Check sheet for the drawn part. Datum: minimum x, y, z corner. Units: mm. A direction names the side the tool comes from. Give positions to 0.01 mm unless a question says otherwise; leave off trailing zeros. Loops run counter-clockwise (first coordinate to the right, second up) from the corner with the lowest first, then second, coordinate; pieces in that order, holes last. Notation, with made-up numbers: (-24, 82) - (-8, 82) arc R24 ccw to (-8, 101) - close; hole circle Ø10 at (62.5, 73). An arc over 180 degrees is marked (long way). Answer in a Markdown table with one row per item.
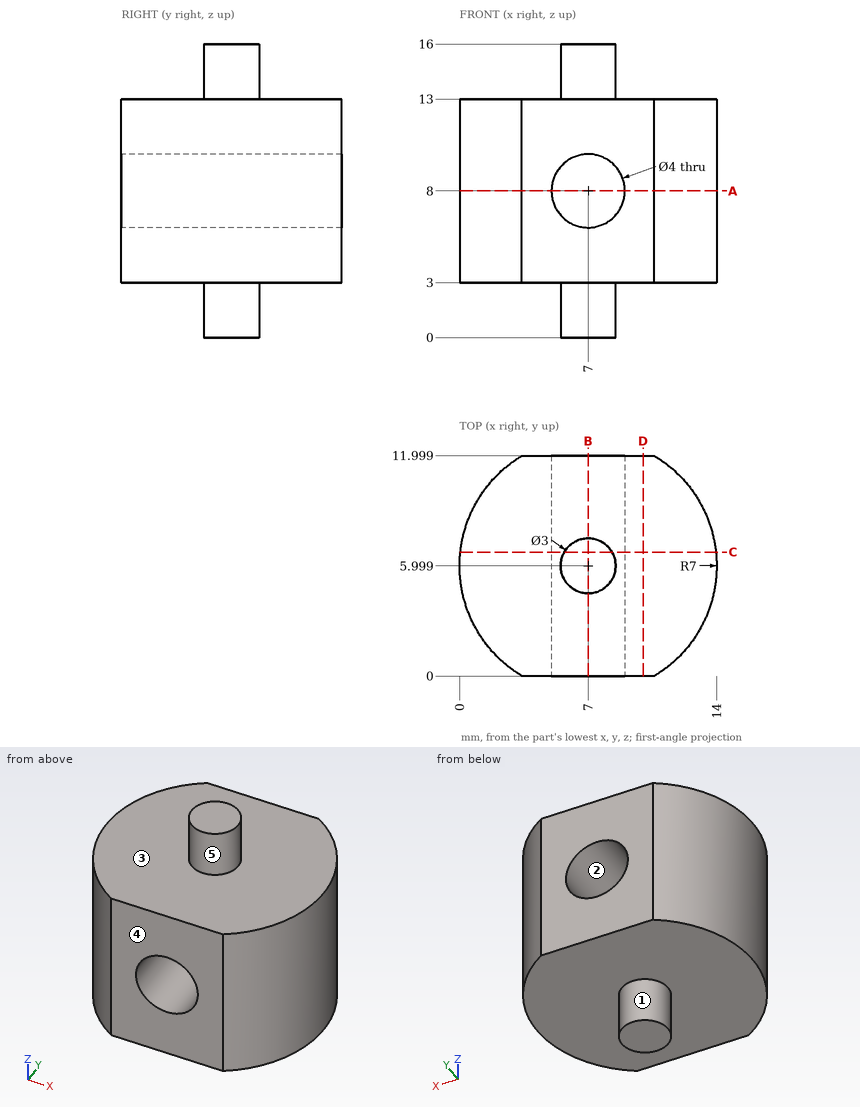
Q1. Draft check along Z on the marked faces 1, 2 and 3. Enter one of: +Z half, -Z half, draft (parallel to the pull), parting line (faces both ways), or undercut.
Completed:
| item | result |
|---|---|
| face 1 | draft |
| face 2 | undercut |
| face 3 | +Z half |
Q2. Sectioned sample at D-D (x = 10). Record the cut outline in (y, z), and give its area (3 significant figures).
Completed:
| item | result |
|---|---|
| outline | (0, 3) - (12, 3) - (12, 13) - (0, 13) - close |
| area | 120 mm^2 |
Q3. Thickness scan on line 1 (Z direction, x = 7, y = 9.5); line 2 (Z direction, x = 2.25, y = 9.75); line 3 (Z direction, x = 8.5, y = 3.75) (1 decimal). Record the ranges inside material, lowest first.
Completed:
| item | result |
|---|---|
| line 1 | 3 to 6, 10 to 13 |
| line 2 | 3 to 13 |
| line 3 | 3 to 6.7, 9.3 to 13 |
Q4. Tool access check on the marked faces 4 and 5. Record the directions out of +Z, -Z, +X, -X, +Y, -Y that give a thin tool (end or side, any length) a straight path to the whole face; none if there is none.
Completed:
| item | result |
|---|---|
| face 4 | +Z, -Z, +X, -X, -Y |
| face 5 | +Z |
Q5. Sectioned sample at C-C (y = 6.75). Record the cut outline in (x, z).
Completed:
| item | result |
|---|---|
| outline | (0.04, 3) - (5.7, 3) - (5.7, 0) - (8.3, 0) - (8.3, 3) - (13.96, 3) - (13.96, 13) - (8.3, 13) - (8.3, 16) - (5.7, 16) - (5.7, 13) - (0.04, 13) - close; hole circle Ø4 at (7, 8) |
Q6. Go/stop test with flat-tipped pins: P1, Ø1, axis at y = 4.5, z = 13, coming from the +X side; P2, Ø5, axis at y = 2, z = 10.5, coming from the -X side; P3, Ø1.5, axis at x = 9.5, y = 4, coming from the -Z side. Record where each tip stops, or that it passes through.
Completed:
| item | result |
|---|---|
| P1 | x = 13.93 |
| P2 | x = 0.16 |
| P3 | z = 3 |
Q7. Sectioned sample at B-B (x = 7). Record the cut outline in (y, z).
Completed:
| item | result |
|---|---|
| outline | (0, 3) - (4.5, 3) - (4.5, 0) - (7.5, 0) - (7.5, 3) - (12, 3) - (12, 6) - (0, 6) - close; (0, 10) - (12, 10) - (12, 13) - (7.5, 13) - (7.5, 16) - (4.5, 16) - (4.5, 13) - (0, 13) - close |
Q8. Sectioned sample at A-A (z = 8). Record the cut outline in (x, y).
Completed:
| item | result |
|---|---|
| outline | (3.39, 0) - (5, 0) - (5, 12) - (3.39, 12) arc R7 ccw to start; (9, 0) - (10.61, 0) arc R7 ccw to (10.61, 12) - (9, 12) - close |
